Input: dimensioned drawing with shaded views. Units: mm. Origin: part minimum x, y, z. A direction names the side the tool comes from. Give positions to 0.01 mm unless a question says otherwise; leave off trailing zeros. Loops run counter-clockwise (first coordinate to the right, second up) from the corner with the lowest first, then second, coordinate; pieces in that order, holes last. Notation, with made-up numbers: M 71.25,58.25 L 97.25,58.25 A11 cw 97.25,66.25 Z; hole C 45,15.25 d2. An arc over 180 degrees is marked long. Use CSV: the item, a comma, the result in double quotes. Start each with the question number.
Q1. Pull-direction query (Y, two-part tool) for the marked faces 1, 2 and 3; classes: released by +Y, released by -Y, zero draft, split by the parting line, or undercut.
Q2. Section A-A, the plane y = 62. Output: boundary loops of the cut face in (x, z), plus the area to 3 significant figures.
Q3. Section C-C, the plane z = 27. Output: boundary loops of the cut face in (x, y), plus the area to 3 significant figures.
Q4. Reachability of the marked faces 4 and 5 from +Z, -Z, +X, -X, +Y, -Y: full face, straight path, thin tool, end or side. Return the list, or none.
Q5. Section D-D, the plane z = 36.5. Output: boundary loops of the cut face in (x, y), plus the area to 3 significant figures.
Q6. Material intervals for line 1 along Y through (x, z) = (35, 27); line 2 along Z through (x, y) = (33.5, 40.5); line 3 along Z through (x, y) = (3.5, 45.5), sorted ascending.
Q7. Section B-B, the plane x = 10.5. Output: boundary loops of the cut face in (y, z), plus the area to 3 significant figures.
Q8. Pin query (flat end, axial travel): pin 1 (7 mm diameter, centred on y = 62, z = 27, fed in from -X). Return the tip coordinate at first contact, or that it passes through.
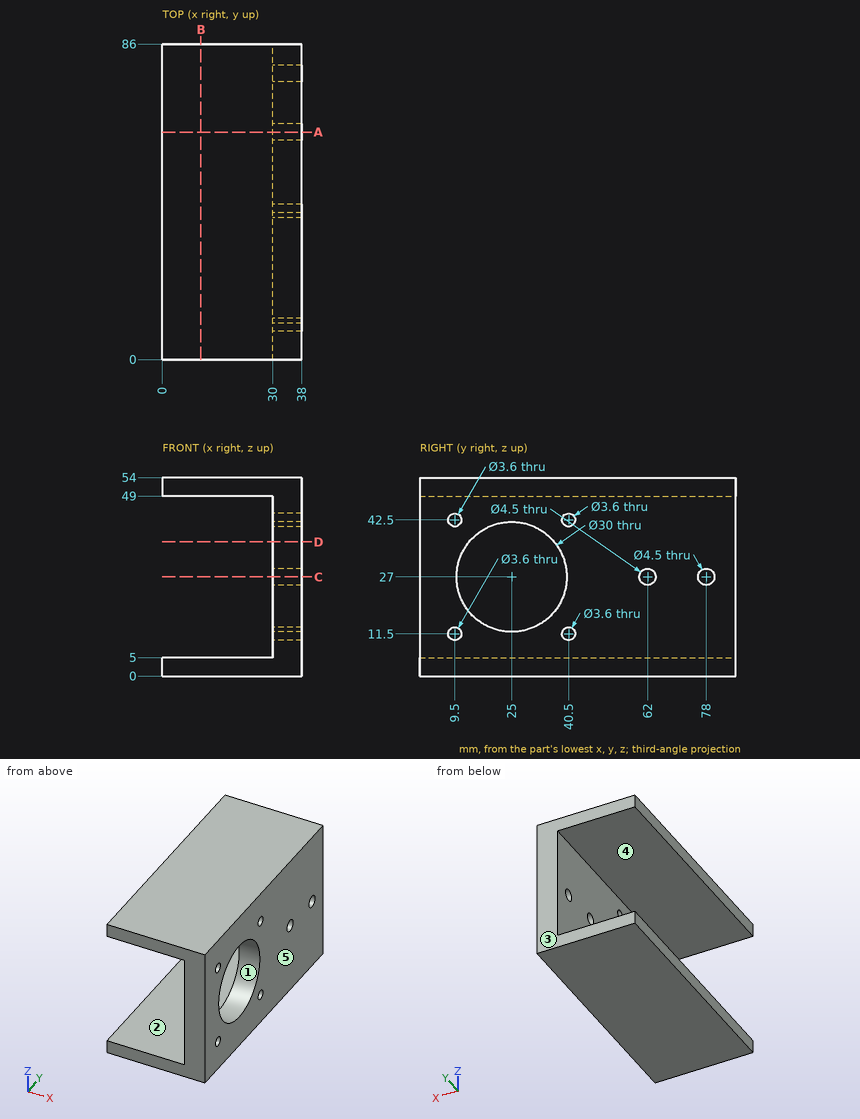
A:
1,face 1,"undercut"
1,face 2,"zero draft"
1,face 3,"released by +Y"
2,outline,"M 0,0 L 38,0 L 38,24.75 L 30,24.75 L 30,5 L 0,5 Z; M 0,49 L 30,49 L 30,29.25 L 38,29.25 L 38,54 L 0,54 Z"
2,area,"696 mm^2"
3,outline,"M 30,0 L 38,0 L 38,10 L 30,10 Z; M 30,40 L 38,40 L 38,59.75 L 30,59.75 Z; M 30,64.25 L 38,64.25 L 38,75.75 L 30,75.75 Z; M 30,80.25 L 38,80.25 L 38,86 L 30,86 Z"
3,area,"376 mm^2"
4,face 4,"-X, +Y, -Y"
4,face 5,"+Z, -Z, +X, +Y, -Y"
5,outline,"M 30,0 L 38,0 L 38,13.39 L 30,13.39 Z; M 30,36.61 L 38,36.61 L 38,86 L 30,86 Z"
5,area,"502 mm^2"
6,line 1,"0 to 10, 40 to 59.75, 64.25 to 75.75, 80.25 to 86"
6,line 2,"0 to 9.7, 13.3 to 40.7, 44.3 to 54"
6,line 3,"0 to 5, 49 to 54"
7,outline,"M 0,0 L 86,0 L 86,5 L 0,5 Z; M 0,49 L 86,49 L 86,54 L 0,54 Z"
7,area,"860 mm^2"
8,pin 1,"x = 30"
